```python
from build123d import *

# Parameters (mm, degrees)
EXTRUDE_1_DEPTH     = 9
SKETCH_3_R          = 2.35
CUT_EXTRUDE_1_DEPTH = 5
SKETCH_4_W          = 2
SKETCH_4_H          = 5
EXTRUDE_3_DEPTH     = 2
EXTRUDE_4_DEPTH     = 3


with BuildPart() as part:
    # Эскиз1 → Бобышка-Вытянуть1 (new body, symmetric)
    with BuildSketch(Plane.XY):
        Polygon((0, 38), (0, 0), (38, 0), (38, 4), (4, 4), (4, 38), align=None)
    extrude(amount=EXTRUDE_1_DEPTH, both=True)

    # Эскиз3 → Вырез-Вытянуть1 (cut, through all)
    with BuildSketch(Plane(origin=(0, 4, 0), x_dir=(1, 0, 0), z_dir=(0, 1, 0))):
        with Locations(Location((14.65, 0, 0), (0, 0, 270))):  # turned: the seam where the file's is
            Circle(SKETCH_3_R)
        with Locations(Location((29.65, 0, 0), (0, 0, 270))):  # turned: the seam where the file's is
            Circle(SKETCH_3_R)
    cut_extrude_1 = extrude(amount=-CUT_EXTRUDE_1_DEPTH, mode=Mode.SUBTRACT)

    # Эскиз4 → Бобышка-Вытянуть3 (add)
    with BuildSketch(Plane.XZ):
        with Locations((1, 0)):
            Rectangle(SKETCH_4_W, SKETCH_4_H)
        with Locations((37, 0)):
            Rectangle(SKETCH_4_W, SKETCH_4_H)
    extrude_3 = extrude(amount=EXTRUDE_3_DEPTH)

    # Зеркальное отражение3: Вырез-Вытянуть1, Бобышка-Вытянуть3 across plane
    add(cut_extrude_1.mirror(Plane(origin=(0, 0, 0), x_dir=(0, 0, 1), z_dir=(-0.707106781, 0.707106781, 0))), mode=Mode.SUBTRACT)
    add(extrude_3.mirror(Plane(origin=(0, 0, 0), x_dir=(0, 0, 1), z_dir=(-0.707106781, 0.707106781, 0))))

    # Эскиз2 → Бобышка-Вытянуть4 (add)
    with BuildSketch(Plane.XY.offset(-9)):
        Polygon((4, 38), (38, 4), (4, 4), align=None)
    extrude(amount=EXTRUDE_4_DEPTH)


solid = part.part
```
Geometry check sheet. Reference: the model listing, model coordinates, mm. A direction names the side the tool comes from. Round coordinates to 2 decimals unless told otherwise and drop trailing zeros. Loops run counter-clockwise (first coordinate to the right, second up) from the corner with the lowest first, then second, coordinate; pieces in that order, holes last. Notation, with made-up numbers: (54.25, 54) - (113.25, 54) arc R18 cw to (113.25, 80) - close; hole circle Ø11 at (52.5, 0.25). An arc over 180 degrees is marked (long way). Write item = value, one per line. Start each with the question number.
1. Depth check by flat-ended pin: pin 1 (6 mm diameter, centred on y = 23, z = -1.5, fed in from -X); pin 2 (0.6 mm diameter, centred on x = 36.5, y = -0.5, fed in from -Z); pin 3 (4 mm diameter, centred on y = 29.65, z = 0, fed in from -X); pin 4 (1.5 mm diameter, centred on x = 19.5, z = 3, fed in from -Y). Enter the tip coordinate at first touch or a pass-through.
2. Set-up check for faces 1 (the face through (1, -1, -2.5)), 2 (the face through (-1, 36, 0)), 3 (the face through (4, 21, 2)), 4 (the face through (2, -1, 0)): record each of +Z, -Z, +X, -X, +Y, -Y from which the full face is reachable in a straight line by a thin tool's end or side.
3. Section check A-A on x = 29.65. Enter the section's corners in (y, z), then the cut area to 4 significant figures.
4. Section check C-C on z = 0. Give the number of separate pieces and of enclosed holes in the cut face, then the cut area to 3 significant figures.
5. Section check B-B on y = 14.65. Enter the section's corners in (x, z), then the cut area to 3 significant figures.
6. Thickness scan on line 1 (X direction, y = 1.6, z = 0); line 2 (X direction, y = 2.5, z = 0). Record the ranges inside material, lowest first.
7. Mould release check, pull along Y, two halves, no side actions. Record for faces 5 (the face through (0, 19, 0)), 6 (the face through (37, -1, -2.5)), 7 (the face through (2, 38, 0)): released by +Y, released by -Y, zero draft, split by the parting line, or undercut.
8. Section check D-D on y = 1. Enter the section's corners in (x, z), then the cut area to 3 significant figures.
Working result:
q1.pin_1 = 0
q1.pin_2 = -2.5
q1.pin_3 = through
q1.pin_4 = 0
q2.face_1 = -Z, +X, -X, -Y
q2.face_2 = +Z, -Z, -X
q2.face_3 = +Z, +X, +Y
q2.face_4 = +Z, -Z, -Y
q3.outline = (0, -9) - (12.35, -9) - (12.35, -6) - (4, -6) - (4, -2.35) - (0, -2.35) - close; (0, 2.35) - (4, 2.35) - (4, 9) - (0, 9) - close
q3.area = 78.25 mm^2
q4.separate_pieces = 5
q4.enclosed_holes = 0
q4.area = 229 mm^2
q5.outline = (0, -9) - (27.35, -9) - (27.35, -6) - (4, -6) - (4, -2.35) - (0, -2.35) - close; (0, 2.35) - (4, 2.35) - (4, 9) - (0, 9) - close
q5.area = 123 mm^2
q6.line_1 = -2 to 12.3, 17 to 27.3, 32 to 38
q6.line_2 = 0 to 12.3, 17 to 27.3, 32 to 38
q7.face_5 = undercut
q7.face_6 = zero draft
q7.face_7 = released by +Y
q8.outline = (-2, -2.5) - (0, -2.5) - (0, -9) - (38, -9) - (38, 9) - (0, 9) - (0, 2.5) - (-2, 2.5) - close; hole circle Ø4.7 at (14.65, 0); hole circle Ø4.7 at (29.65, 0)
q8.area = 659 mm^2
